Could you check a few things on this model? Use its own coordinates, in mm. A direction names the side the tool comes from. Coordinates: 2 decimals unless noted, no trailing zeros. Write each loop counter-clockwise with the first axis right and the second up, starting at its lowest first coordinate (ties: lowest second). Pieces come first, ordered by that corner, then holes.
```python
from build123d import *

# Parameters (mm, degrees)
SKETCH1_W               = 85
SKETCH1_H               = 15
BOSS_EXTRUDE1_DEPTH     = 25
SKETCH2_W               = 3.4
SKETCH2_H               = 7.9
BOSS_EXTRUDE2_DEPTH     = 2.8
CUT_EXTRUDE2_DEPTH      = 90.744582009
CUT_EXTRUDE2_DEPTH_BACK = 90.744582009
SKETCH5_R               = 1.651
CUT_EXTRUDE3_DEPTH      = 9.525


with BuildPart() as part:
    # Sketch1 → Boss-Extrude1 (new body)
    with BuildSketch(Plane(origin=(0, 0, 0), x_dir=(1, 0, 0), z_dir=(0, 1, 0))):
        Rectangle(SKETCH1_W, SKETCH1_H)
    extrude(amount=BOSS_EXTRUDE1_DEPTH)

    # Sketch2 → Boss-Extrude2 (add)
    with BuildSketch(Plane(origin=(0, 25, 0), x_dir=(1, 0, 0), z_dir=(0, 1, 0))):
        with Locations((-40.8, 0)):
            Rectangle(SKETCH2_W, SKETCH2_H)
        with Locations((40.8, 0)):
            Rectangle(SKETCH2_W, SKETCH2_H)
    extrude(amount=BOSS_EXTRUDE2_DEPTH)

    # Sketch3 → Cut-Extrude2 (cut, two sides: drawn at the far end of the back side and taken through both)
    with BuildSketch(Plane(origin=(42.5, 0, 0), x_dir=(0, 0, -1), z_dir=(1, 0, 0)).offset(-CUT_EXTRUDE2_DEPTH_BACK)):
        Polygon((-2, 0), (2, 0), (2, 6), (4.25, 6), (4.25, 10), (-4.25, 10), (-4.25, 6), (-2, 6), align=None)
    extrude(amount=CUT_EXTRUDE2_DEPTH + CUT_EXTRUDE2_DEPTH_BACK, mode=Mode.SUBTRACT)

    # Sketch5 → Cut-Extrude3 (cut)
    with BuildSketch(Plane(origin=(0, 25, 0), x_dir=(1, 0, 0), z_dir=(0, 1, 0))):
        with Locations(Location((33, 0, 0), (0, 0, 270))):
            Circle(SKETCH5_R)
        with Locations(Location((-33, 0, 0), (0, 0, 270))):
            Circle(SKETCH5_R)
    extrude(amount=-CUT_EXTRUDE3_DEPTH, mode=Mode.SUBTRACT)


solid = part.part
```
Item 1: I want a section at C-C, the plane z = 0. List the corners of the cut face in (x, y) for me (3 decimals), then the cut area to 3 significant figures.
Item 2: Will these pins go through, and if not, where does the flat tip stop? pin 1 Ø1.4 at (x, y) = (-40, 26) entering from -Z; pin 2 Ø2 at (x, z) = (-33, 0) entering from +Y (3 decimals); pin 3 Ø7.5 at (x, z) = (20.5, 0) entering from +Y.
Item 3: I want a section at A-A, the plane y = 25.75. List the corners of the cut face in (x, z) for me, then the cut area to 3 significant figures.
Item 4: Which directions (+Z, -Z, +X, -X, +Y, -Y) give clear straight access to the entire face, cutting with the end or side of a thin tool? Please do faces 4 (the flat face through (39.1, 26, 0)), 5 (the flat face through (-41, 26, -3.95)), 6 (the flat face through (-41, 26, 3.95)).
Item 5: I want a section at B-B, the plane x = -27.5. List the corners of the cut face in (y, z) for me.
Item 6: If I drill on line 1 along X through (y, z) = (19.5, 0); line 2 along Y through (x, z) = (11.5, -3.25); line 3 along Z through (x, y) = (37, 6.5), over which ranges is the centre line in solid material (lowest first)?
Item 7: If we mould it in two halves opening along Z, with no side actions, what happens to faces 1 (the flat face through (-42.5, 14, 0)), 2 (the cylindrical face through (-31.363, 20.304, -0.215)), 3 (the flat face through (41, 26, 3.95))? For each: released by +Z, released by -Z, zero draft, split by the parting line, or undercut.
Item 8: I want a section at D-D, the plane z = 5.5. List the corners of the cut face in (x, y) for me.
Taken from the geometry:
1. outline: (-42.5, 10) - (42.5, 10) - (42.5, 27.8) - (39.1, 27.8) - (39.1, 25) - (34.651, 25) - (34.651, 15.475) - (31.349, 15.475) - (31.349, 25) - (-31.349, 25) - (-31.349, 15.475) - (-34.651, 15.475) - (-34.651, 25) - (-39.1, 25) - (-39.1, 27.8) - (-42.5, 27.8) - close
1. area: 1,230 mm2
2. pin 1: stops at z = -3.95
2. pin 2: stops at y = 15.475
2. pin 3: stops at y = 25
3. outline: (-42.5, -3.95) - (-39.1, -3.95) - (-39.1, 3.95) - (-42.5, 3.95) - close; (39.1, -3.95) - (42.5, -3.95) - (42.5, 3.95) - (39.1, 3.95) - close
3. area: 53.7 mm2
4. face 4: +Z, -Z, +Y
4. face 5: -Z, +X, -X, +Y
4. face 6: +Z, +X, -X, +Y
5. outline: (0, -7.5) - (25, -7.5) - (25, 7.5) - (0, 7.5) - (0, 2) - (6, 2) - (6, 4.25) - (10, 4.25) - (10, -4.25) - (6, -4.25) - (6, -2) - (0, -2) - close
6. line 1: x = -42.5 to -34.65, -31.35 to 31.35, 34.65 to 42.5
6. line 2: y = 0 to 6, 10 to 25
6. line 3: z = -7.5 to -4.25, 4.25 to 7.5
7. face 1: zero draft
7. face 2: undercut
7. face 3: released by +Z
8. outline: (-42.5, 0) - (42.5, 0) - (42.5, 25) - (-42.5, 25) - close
